The listing builds one solid part. Answer for the finished solid, in the listing's coordinates (mm). Face numbers are marked on the shaded views. Give positions to 0.01 mm unless a question says otherwise; leave off trailing zeros. Loops run counter-clockwise (first coordinate to the right, second up) from the corner with the lowest first, then second, coordinate; pieces in that order, holes last. Notation, with made-up numbers: M 40,-2.5 L 50,-2.5 A28 ccw 50,34.5 Z; hole C 65,-5 d4. An arc over 180 degrees is marked long. One line per item, written item: value. Start each with the question number.
Q1. A cutting plane is placed at C-C, the plane z = 30.5. Determine the outline of the cut face in (x, y).
Q2. Consider L1, parallel to Y at x = 192.5, z = 37; L2, parallel to Z at x = 352, y = 7; L3, parallel to Z at x = 557, y = 25. Determine where each line is inside the solid, lowest interval first.
Q3. A cutting plane is placed at B-B, the plane y = 25.5. Determine the outline of the cut face in (x, z).
Q4. The mould has two halves that part along Z. Classify the marked faces 1 and 2: +Z half, -Z half, draft (parallel to the pull), parting line (faces both ways), or undercut.
Q5. A flat-ended cylindrical pin translates along its axis: pin 1 (2 mm diameter, centred on x = 194, z = 58, fed in from +Y). Find the tip coordinate at first contact, or state that the pin passes through.
Q6. A cutting plane is placed at A-A, the plane x = 292. Determine the outline of the cut face in (y, z), and give its area (3 significant figures).
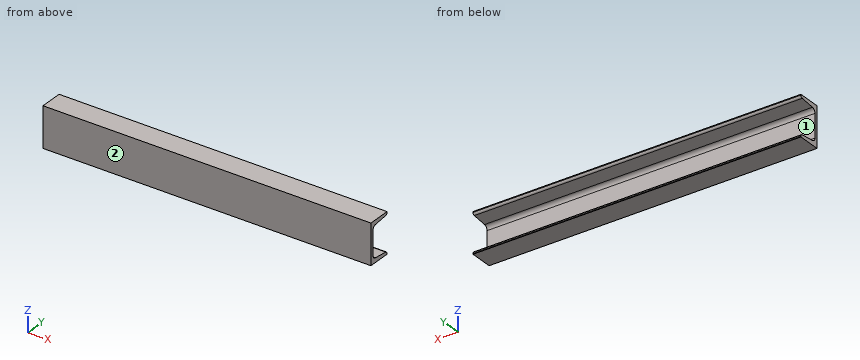
from build123d import *

# Parameters (mm, degrees)
CANAL_C_80_X_8_1_DEPTH = 650


with BuildPart() as part:
    # Sketch15 → Canal c 80 X 8(1) (new body)
    with BuildSketch(Plane.YZ):
        with BuildLine():
            Line((45, 80), (0, 80))
            Line((0, 80), (0, 0))
            Line((0, 0), (45, 0))
            Line((45, 0), (45, 1.822575175))
            ThreePointArc((45, 1.822575175), (43.972579302, 4.499097601), (41.418113853, 5.800662757))
            Line((41.418113853, 5.800662757), (12.663772294, 8.822865837))
            ThreePointArc((12.663772294, 8.822865837), (7.554841396, 11.425996149), (5.5, 16.779041))
            Line((5.5, 16.779041), (5.5, 63.220959))
            ThreePointArc((5.5, 63.220959), (7.554841396, 68.574003851), (12.663772294, 71.177134163))
            Line((12.663772294, 71.177134163), (41.418113853, 74.199337243))
            ThreePointArc((41.418113853, 74.199337243), (43.972579302, 75.500902399), (45, 78.177424825))
            Line((45, 78.177424825), (45, 80))
        make_face()
    extrude(amount=CANAL_C_80_X_8_1_DEPTH)


solid = part.part
Answer block:
1. outline: M 0,0 L 650,0 L 650,5.5 L 0,5.5 Z
2. L1: 0 to 5.5
2. L2: 0 to 12.12, 67.88 to 80
2. L3: 0 to 7.53, 72.47 to 80
3. outline: M 0,0 L 650,0 L 650,7.47 L 0,7.47 Z; M 0,72.53 L 650,72.53 L 650,80 L 0,80 Z
4. face 1: undercut
4. face 2: draft
5. pin 1: y = 5.5
6. outline: M 0,0 L 45,0 L 45,1.82 A4 ccw 41.42,5.8 L 12.66,8.82 A8 cw 5.5,16.78 L 5.5,63.22 A8 cw 12.66,71.18 L 41.42,74.2 A4 ccw 45,78.18 L 45,80 L 0,80 Z
6. area: 1,050 mm^2
